Model file for the job. Use its own axes, mm. Face numbers are marked on the shaded views. A direction names the side the tool comes from. Give positions to 0.01 mm unless a question says otherwise; leave off trailing zeros. Write each loop counter-clockwise with the first axis right and the second up, starting at its lowest first coordinate (ties: lowest second). Pieces come first, ordered by that corner, then holes. Notation, with made-up numbers: M 68.5,86.25 L 72.5,86.25 A13 cw 72.5,99.25 Z; hole C -2.75,30 d11. An arc over 180 degrees is marked long. Answer as a JSON object with one key per item and string values. Group by question number.
```python
from build123d import *

# Parameters (mm, degrees)
F0_W     = 800
F0_H     = 400
F1_DEPTH = 40
F3_DEPTH = 800.001
F5_DEPTH = 20
F8_W     = 800
F8_H     = 360
F9_DEPTH = 100.001


with BuildPart() as f1:
    # F0 (on Top) → F1 (new body, symmetric)
    with BuildSketch(Plane.XY):
        Rectangle(F0_W, F0_H)
    extrude(amount=F1_DEPTH, both=True)

    # F2 (on face) → F3 (cut, through all)
    with BuildSketch(Plane.YZ.offset(400)):
        Polygon((-180, -20), (-180, -20.0497749922), (-179.5264225832, -20), align=None)
        Polygon((-200, -2.0416941063), (200, 40), (-200, 40), align=None)
    extrude(amount=-F3_DEPTH, mode=Mode.SUBTRACT)

    # F4 (on face) → F5 (join)
    with BuildSketch(Plane.YZ.offset(400)):
        Polygon((200, 40), (-200, -2.0416941063), (-200, -40), (200, -40), align=None)
        Polygon((-179.5264225832, -20), (-180, -20.0497749922), (-180, -20), align=None, mode=Mode.SUBTRACT)
        Polygon((-180, -20), (-180, -20.0497749922), (-179.5264225832, -20), align=None)
    extrude(amount=F5_DEPTH)

    # F6: F1 across plane


with BuildPart() as f1_1:
    add(f1.part)
    add(f1.part.mirror(Plane.YZ))

    # F8 (on offset) → F9 (cut, through all)
    with BuildSketch(Plane(origin=(0, 0, -60), x_dir=(1, 0, 0), z_dir=(0, 0, -1))):
        Rectangle(F8_W, F8_H)
    extrude(amount=-F9_DEPTH, mode=Mode.SUBTRACT)


solid = f1_1.part
```
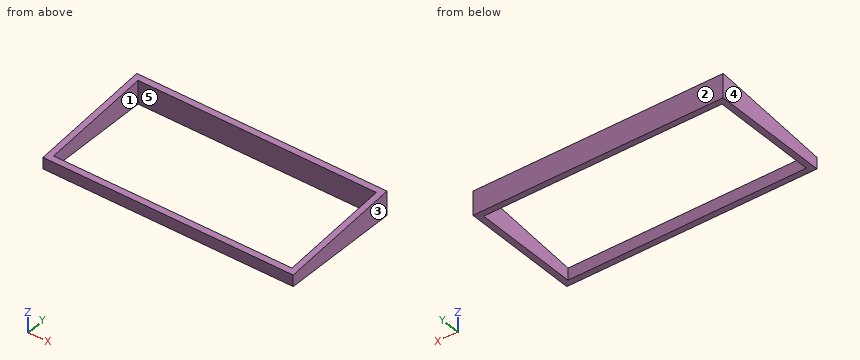
Q1. 3-axis set-ups, long thin cutter, end or side, ignore diameter. For the marked faces 1 and 2: which of +Z, -Z, +X, -X, +Y, -Y reach the whole face in a straight line?
Q2. Slice it at C-C, the plane y = -15. Write the cut outline in (x, z).
Q3. Slice it at D-D, the plane z = 23. Write the cut outline in (x, y).
Q4. Slice it at A-A, the plane x = -148.5. Write the cut outline in (y, z), then the cut area to 3 significant figures.
Q5. Wall check: L1, parallel to Y at x = 182, z = -32; L2, parallel to X at y = 99.5, z = -13; L3, parallel to Y at x = 15, z = 11. Give the ranges that are in metal, low to high.
Q6. Slice it at B-B, the plane z = -28. Write the cut outline in (x, y).
Q7. Two-plate mould, pull along X, no slides. Class the marked faces 3, 4 and 5: +X half, -X half, draft (parallel to the pull), parting line (faces both ways), or undercut.
Solved:
{
 "1": {"face 1": "+Z, -Z", "face 2": "+Z, -Z, +X, -X, +Y"},
 "2": {"outline": "M -420,-40 L -400,-40 L -400,17.4 L -420,17.4 Z; M 400,-40 L 420,-40 L 420,17.4 L 400,17.4 Z"},
 "3": {"outline": "M -420,38.26 L -400,38.26 L -400,180 L 400,180 L 400,38.26 L 420,38.26 L 420,200 L -420,200 Z"},
 "4": {"outline": "M -200,-40 L -180,-40 L -180,0.06 L -200,-2.04 Z; M 180,-40 L 200,-40 L 200,40 L 180,37.9 Z", "area": "2,360 mm²"},
 "5": {"L1": "y = -200 to -180, 180 to 200", "L2": "x = -420 to -400, 400 to 420", "L3": "y = 180 to 200"},
 "6": {"outline": "M -420,-200 L 420,-200 L 420,200 L -420,200 Z; hole M -400,-180 L 400,-180 L 400,180 L -400,180 Z"},
 "7": {"face 3": "+X half", "face 4": "-X half", "face 5": "undercut"}
}
